Geometry: final body of the model. Coordinates: model frame, mm. Face numbers are marked on the shaded views. A direction names the side the tool comes from. Give positions to 0.01 mm unless a question says otherwise; leave off trailing zeros. Order: outer loops, then holes, each group sorted by start corner. A loop starts at its lowest first (then second) coordinate and runs counter-clockwise, first axis right, second up. Notation, with made-up numbers: (-19, -28) -> (1, -28) arc R24 ccw to (1, -12) -> close; hole circle Ø4 at (57, 82.25). An arc over 180 degrees is marked (long way). One line per question, with ' | ' between items.
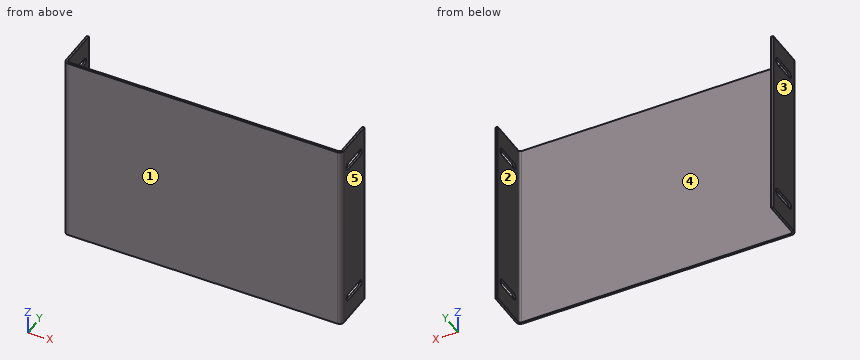
from build123d import *

# Parameters (mm, degrees)
SKETCH1_W               = 94.2208
SKETCH1_H               = 67.5
BASE_FLANGE1_DEPTH      = 0.7366
EDGE_FLANGE1_DEPTH      = 67.5
EDGE_FLANGE1_BEND_DEPTH = 67.5
CUT_EXTRUDE1_DEPTH      = 105.682033016


# Sheet-metal steps are written as plain solids
with BuildPart() as part:
    # Sketch1 → Base-Flange1 (new body)
    with BuildSketch(Plane(origin=(0, 0, 0), x_dir=(1, 0, 0), z_dir=(0, 1, 0))):
        with Locations((0, -1.046060421)):
            Rectangle(SKETCH1_W, SKETCH1_H)
    extrude(amount=-BASE_FLANGE1_DEPTH)

    # Edge-Flange1 section (across the edge) → Edge-Flange1 (add)
    with BuildSketch(Plane(origin=(48.1104, 0, 34.796060421), x_dir=(-1, 0, 0), z_dir=(0, 0, -1))):
        with BuildLine():
            Line((-0.7366, 0.7366), (-0.7366, 14.2634))
            Line((-0.7366, 14.2634), (0, 14.2634))
            Line((0, 14.2634), (0, 0.7366))
            ThreePointArc((0, 0.7366), (0.215745145, 0.215745145), (0.7366, 0))
            Line((0.7366, 0), (1, 0))
            Line((1, 0), (1, -0.7366))
            Line((1, -0.7366), (0.7366, -0.7366))
            ThreePointArc((0.7366, -0.7366), (-0.30510971, -0.30510971), (-0.7366, 0.7366))
        make_face()
    extrude(amount=EDGE_FLANGE1_DEPTH)

    # Edge-Flange1 section 2 (across the edge) → Edge-Flange1 bend (add)
    with BuildSketch(Plane(origin=(-48.1104, 0, -32.703939579), x_dir=(1, 0, 0), z_dir=(0, 0, 1))):
        with BuildLine():
            Line((-0.7366, 0.7366), (-0.7366, 14.2634))
            Line((-0.7366, 14.2634), (0, 14.2634))
            Line((0, 14.2634), (0, 0.7366))
            ThreePointArc((0, 0.7366), (0.215745145, 0.215745145), (0.7366, 0))
            Line((0.7366, 0), (1, 0))
            Line((1, 0), (1, -0.7366))
            Line((1, -0.7366), (0.7366, -0.7366))
            ThreePointArc((0.7366, -0.7366), (-0.30510971, -0.30510971), (-0.7366, 0.7366))
        make_face()
    extrude(amount=EDGE_FLANGE1_BEND_DEPTH)

    # Sketch13 → Cut-Extrude1 (cut, through all)
    with BuildSketch(Plane.ZY.offset(48.847)):
        with BuildLine():
            Line((28.046060421, 11.2634), (28.046060421, 3.7634))
            ThreePointArc((28.046060421, 3.7634), (26.796060421, 2.5134), (25.546060421, 3.7634))
            Line((25.546060421, 3.7634), (25.546060421, 11.2634))
            ThreePointArc((25.546060421, 11.2634), (26.796060421, 12.5134), (28.046060421, 11.2634))
        make_face()
        with BuildLine():
            Line((-23.453939579, 11.2634), (-23.453939579, 3.7634))
            ThreePointArc((-23.453939579, 3.7634), (-24.703939579, 2.5134), (-25.953939579, 3.7634))
            Line((-25.953939579, 3.7634), (-25.953939579, 11.2634))
            ThreePointArc((-25.953939579, 11.2634), (-24.703939579, 12.5134), (-23.453939579, 11.2634))
        make_face()
    extrude(amount=-CUT_EXTRUDE1_DEPTH, mode=Mode.SUBTRACT)


solid = part.part
1) Section A-A on y = 6. Return loops of the section in (x, z).
Check result:
outline: (-48.85, -32.7) -> (-48.11, -32.7) -> (-48.11, -25.95) -> (-48.85, -25.95) -> close; (-48.85, -23.45) -> (-48.11, -23.45) -> (-48.11, 25.55) -> (-48.85, 25.55) -> close; (-48.85, 28.05) -> (-48.11, 28.05) -> (-48.11, 34.8) -> (-48.85, 34.8) -> close; (48.11, -32.7) -> (48.85, -32.7) -> (48.85, -25.95) -> (48.11, -25.95) -> close; (48.11, -23.45) -> (48.85, -23.45) -> (48.85, 25.55) -> (48.11, 25.55) -> close; (48.11, 28.05) -> (48.85, 28.05) -> (48.85, 34.8) -> (48.11, 34.8) -> close
2) Section B-B on z = -18. Return loops of the section in (x, y), plus the area to 3 significant figures.
Check result:
outline: (-48.85, 0.74) arc R1.47 ccw to (-47.37, -0.74) -> (47.37, -0.74) arc R1.47 ccw to (48.85, 0.74) -> (48.85, 14.26) -> (48.11, 14.26) -> (48.11, 0.74) arc R0.74 cw to (47.37, 0) -> (-47.37, 0) arc R0.74 cw to (-48.11, 0.74) -> (-48.11, 14.26) -> (-48.85, 14.26) -> close | area: 92.3 mm^2
3) Material intervals for probe 1 along X at (y, z) = (6.75, 31); probe 2 along Y at (x, z) = (-25, 24.5), sorted ascending. Write a range as from..to.
Check result:
probe 1: x = -48.85..-48.11, 48.11..48.85 | probe 2: y = -0.74..0
4) Section C-C on x = 25. Return loops of the section in (y, z).
Check result:
outline: (-0.74, -32.7) -> (0, -32.7) -> (0, 34.8) -> (-0.74, 34.8) -> close
5) Contact query for flat-ended pins moving along their axis: pin 1 Ø8 at (x, y) = (-17.5, 7.5) entering from -Z; pin 2 Ø10 at (x, z) = (8.5, 9) entering from +Y. Output: stop coordinate, or through.
Check result:
pin 1: passes through | pin 2: stops at y = 0
6) Set-up query: the marked faces 4 and 5. Return all of +Z, -Z, +X, -X, +Y, -Y with unobstructed straight access to the full face (end or side cutting, diameter ignored); none if empty.
Check result:
face 4: +Z, -Z, +Y | face 5: +Z, -Z, +X, +Y, -Y
7) Pull-direction query (X, two-part tool) for the marked faces 1, 2 and 3; classes: +X half, -X half, draft (parallel to the pull), parting line (faces both ways), or undercut.
Check result:
face 1: draft | face 2: undercut | face 3: -X half
